Drawing for the job (mm, zero at the part's lowest x, y, z). A direction names the side the tool comes from. Coordinates: 2 decimals unless noted, no trailing zeros. Order: outer loops, then holes, each group sorted by start corner. A loop starts at its lowest first (then second) coordinate and runs counter-clockwise, first axis right, second up.
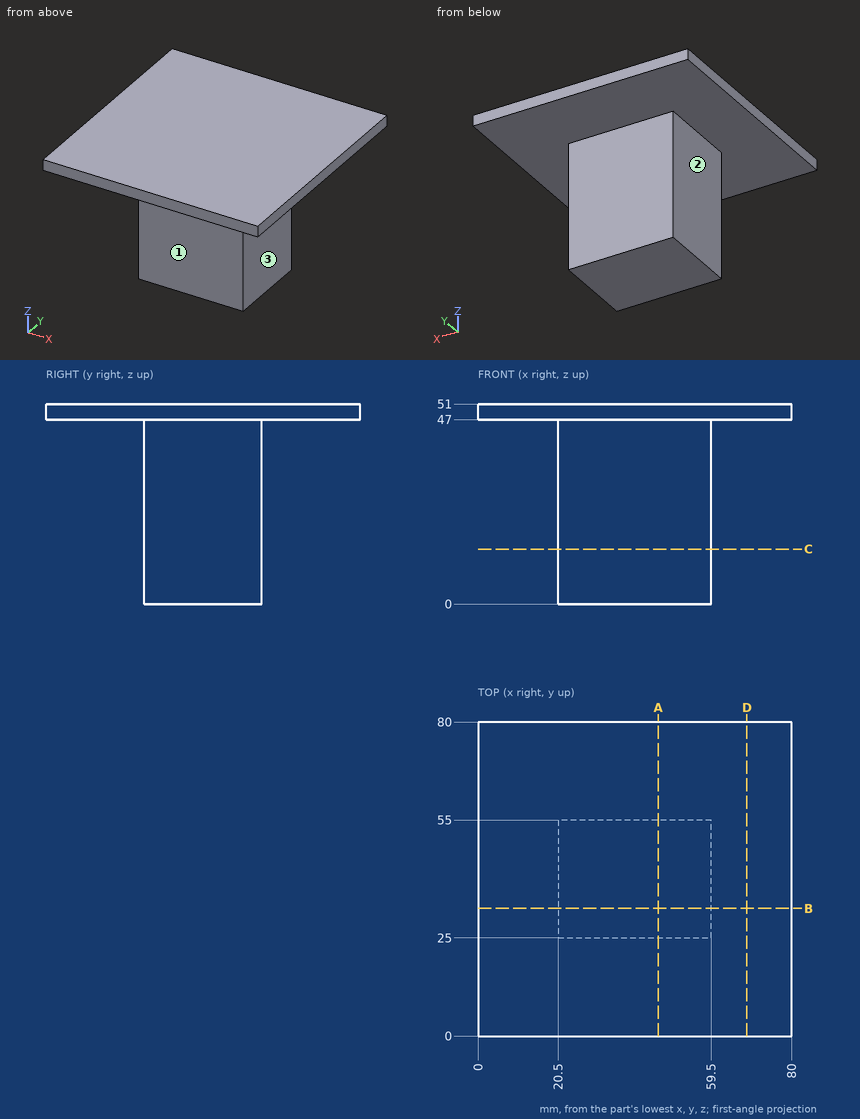
1) Slice it at A-A (x = 46). List the corners of the cut face in (y, z).
2) Which spindle directions (+Z, -Z, +X, -X, +Y, -Y) get a long thin tool onto all of the face, cutting with end or side? Do the marked faces 1, 2 and 3. Say none if no direction does.
3) Slice it at C-C (z = 14). List the corners of the cut face in (x, y), plus the area to 3 significant figures.
4) Slice it at D-D (x = 68.5). List the corners of the cut face in (y, z), plus the area to 3 significant figures.
5) Pin check, flat tips, straight feed: P1, Ø11.5, axis at x = 48, z = 26, coming from the -Y side; P2, Ø2, axis at y = 54.5, z = 7, coming from the -X side; P3, Ø8, axis at x = 20, z = 11, coming from the +Y side; P4, Ø10, axis at x = 14.5, z = 18, coming from the -Y side. Stop position of each tip, or through.
6) Slice it at B-B (y = 32.5). List the corners of the cut face in (x, z), plus the area to 3 significant figures.
7) Drill centre lines: probe 1 along X at (y, z) = (47.5, 5.5); probe 2 along Y at (x, z) = (41, 9); probe 3 along Z at (x, y) = (43.5, 4.5). Where is each one in solid material? Low to high.
Worked out:
1. outline: (0, 47) - (25, 47) - (25, 0) - (55, 0) - (55, 47) - (80, 47) - (80, 51) - (0, 51) - close
2. face 1: -Z, +X, -X, -Y
2. face 2: -Z, -X, +Y, -Y
2. face 3: -Z, +X, +Y, -Y
3. outline: (20.5, 25) - (59.5, 25) - (59.5, 55) - (20.5, 55) - close
3. area: 1,170 mm2
4. outline: (0, 47) - (80, 47) - (80, 51) - (0, 51) - close
4. area: 320 mm2
5. P1: stops at y = 25
5. P2: stops at x = 20.5
5. P3: stops at y = 55
5. P4: passes through
6. outline: (0, 47) - (20.5, 47) - (20.5, 0) - (59.5, 0) - (59.5, 47) - (80, 47) - (80, 51) - (0, 51) - close
6. area: 2,150 mm2
7. probe 1: x = 20.5 to 59.5
7. probe 2: y = 25 to 55
7. probe 3: z = 47 to 51
